from build123d import *

# Parameters (mm, degrees)
F0_W     = 30.2
F0_H     = 15.5
F1_DEPTH = 82
F2_T     = -1
F3_SIZE  = 1
F4_SIZE  = 1


with BuildPart() as f1:
    # F0 (on Top) → F1 (new body)
    with BuildSketch(Plane.XY):
        with Locations((4.6029518125, -7.7385634869)):
            Rectangle(F0_W, F0_H)
    extrude(amount=F1_DEPTH)

    # F2
    f2_openings = [f1.faces().sort_by_distance(p)[0] for p in [
        (4.602952, -7.738563, 82),
    ]]
    offset(amount=F2_T, openings=f2_openings)

    # F3
    f3_edges = [f1.edges().sort_by_distance(p)[0] for p in [
        (19.702952, 0.011437, 41),
        (19.702952, -15.488563, 41),
        (-10.497048, 0.011437, 41),
        (-10.497048, -15.488563, 41),
        (4.602952, 0.011437, 0),
        (19.702952, -7.738563, 0),
        (4.602952, -15.488563, 0),
        (-10.497048, -7.738563, 0),
    ]]
    chamfer(f3_edges, length=F3_SIZE)

    # F4
    f4_edges = [f1.edges().sort_by_distance(p)[0] for p in [
        (-9.497048, -0.988563, 41.5),
        (18.702952, -0.988563, 41.5),
        (18.702952, -14.488563, 41.5),
        (-9.497048, -14.488563, 41.5),
    ]]
    chamfer(f4_edges, length=F4_SIZE)


solid = f1.part
Work out the finished part from the listing and answer in its coordinate system (mm). A direction names the side the tool comes from. Round coordinates to 2 decimals unless told otherwise and drop trailing zeros. Write each loop counter-clockwise with the first axis right and the second up, starting at its lowest first coordinate (ties: lowest second). Pieces come first, ordered by that corner, then holes.
1) Straight lines are drawn through the part: line 1 (Y direction, x = -2, z = 70.5); line 2 (X direction, y = -7, z = 14.5); line 3 (Z direction, x = -2.5, y = -11). For each, find the intervals that lie inside material, in ascending order.
2) The mould has two halves that part along X. Classify faces 1 (the flat face through (-9.497, -8, 41)), 2 (the flat face through (19.703, -8, 41)), 3 (the flat face through (3, -15, 82)), 4 (the flat face through (18.703, -8, 41)): pulls with the +X half, pulls with the -X half, needs draft (parallel to the pull), parting line crosses it, or undercut.
3) Given pin 1 Ø5 at (x, y) = (15, -5) entering from +Z, flat-ended and moving along its own axis, determine where the tip first touches the part or whether it passes through.
4) A cutting plane is placed at B-B (x = -1). Give the vertices of the cut face in (y, z), plus the area to 4 significant figures.
5) A tool of negligible diameter and unlimited length cuts with its end or side. For faces 5 (the flat face through (4, -0.989, 41)), 6 (the flat face through (4, -8, 0)), from which of +Z, -Z, +X, -X, +Y, -Y can it reach the whole face along a straight path? Write none if from no direction.
6) A cutting plane is placed at A-A (z = 20). Give the vertices of the cut face in (x, y).
7) A cutting plane is placed at C-C (y = -7.75). Give the vertices of the cut face in (x, z), plus the area to 3 significant figures.
Completed:
1. line 1: y = -15.49 to -14.49, -0.99 to 0.01
1. line 2: x = -10.5 to -9.5, 18.7 to 19.7
1. line 3: z = 0 to 1
2. face 1: undercut
2. face 2: pulls with the +X half
2. face 3: needs draft
2. face 4: undercut
3. pin 1: stops at z = 1
4. outline: (-15.49, 1) - (-14.49, 0) - (-0.99, 0) - (0.01, 1) - (0.01, 82) - (-0.99, 82) - (-0.99, 1) - (-14.49, 1) - (-14.49, 82) - (-15.49, 82) - close
4. area: 176.5 mm2
5. face 5: +Z
5. face 6: -Z, +X, -X, +Y, -Y
6. outline: (-10.5, -14.49) - (-9.5, -15.49) - (18.7, -15.49) - (19.7, -14.49) - (19.7, -0.99) - (18.7, 0.01) - (-9.5, 0.01) - (-10.5, -0.99) - close; hole (-9.5, -13.49) - (-8.5, -14.49) - (17.7, -14.49) - (18.7, -13.49) - (18.7, -1.99) - (17.7, -0.99) - (-8.5, -0.99) - (-9.5, -1.99) - close
7. outline: (-10.5, 1) - (-9.5, 0) - (18.7, 0) - (19.7, 1) - (19.7, 82) - (18.7, 82) - (18.7, 1) - (-9.5, 1) - (-9.5, 82) - (-10.5, 82) - close
7. area: 191 mm2
